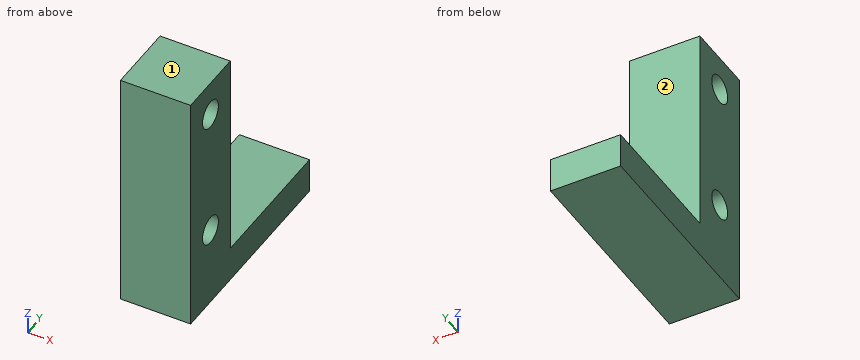
```python
from build123d import *

# Parameters (mm, degrees)
PAD_DEPTH    = 20
SKETCH001_R  = 4
POCKET_DEPTH = 20


with BuildPart() as part:
    # Sketch → Pad (new body)
    with BuildSketch(Plane.YZ):
        Polygon((-10, 35), (-10, -35), (50, -35), (50, -25), (10, -25), (10, 35), align=None)
    extrude(amount=PAD_DEPTH)

    # Sketch001 → Pocket (cut)
    with BuildSketch(Plane.YZ.offset(20)):
        with Locations((0, 25)):
            Circle(SKETCH001_R)
        with Locations((0, -12)):
            Circle(SKETCH001_R)
    extrude(amount=-POCKET_DEPTH, mode=Mode.SUBTRACT)


solid = part.part
```
Verification items for the finished model (mm, model axes). Face numbers are marked on the shaded views. A direction names the side the tool comes from. Give positions to 0.01 mm unless a question says otherwise; leave off trailing zeros. Loops run counter-clockwise (first coordinate to the right, second up) from the corner with the lowest first, then second, coordinate; pieces in that order, holes last.
1. Section check A-A, the plane y = 0. Enter the section's corners in (x, z).
2. Section check C-C, the plane x = 2.25. Enter the section's corners in (y, z).
3. Section check B-B, the plane z = 25. Enter the section's corners in (x, y).
4. Go/stop test with flat-tipped pins: pin 1 Ø6 at (x, y) = (11, 34) entering from +Z; pin 2 Ø10.5 at (y, z) = (0, -12) entering from -X; pin 3 Ø10 at (x, z) = (13, 7) entering from +Y. Record where each tip stops, or that it passes through.
5. Section check D-D, the plane z = 10.5. Enter the section's corners in (x, y), then the cut area to 3 significant figures.
6. Thickness scan on line 1 (Z direction, x = 15.5, y = 0); line 2 (Z direction, x = 13.25, y = -2.5); line 3 (Z direction, x = 4.25, y = 14). Record the ranges inside material, lowest first.
7. Set-up check for the marked faces 1 and 2: record each of +Z, -Z, +X, -X, +Y, -Y from which the full face is reachable in a straight line by a thin tool's end or side.
Geometry says:
1. outline: (0, -35) - (20, -35) - (20, -16) - (0, -16) - close; (0, -8) - (20, -8) - (20, 21) - (0, 21) - close; (0, 29) - (20, 29) - (20, 35) - (0, 35) - close
2. outline: (-10, -35) - (50, -35) - (50, -25) - (10, -25) - (10, 35) - (-10, 35) - close; hole circle Ø8 at (0, -12); hole circle Ø8 at (0, 25)
3. outline: (0, -10) - (20, -10) - (20, -4) - (0, -4) - close; (0, 4) - (20, 4) - (20, 10) - (0, 10) - close
4. pin 1: stops at z = -25
4. pin 2: stops at x = 0
4. pin 3: stops at y = 10
5. outline: (0, -10) - (20, -10) - (20, 10) - (0, 10) - close
5. area: 400 mm2
6. line 1: z = -35 to -16, -8 to 21, 29 to 35
6. line 2: z = -35 to -15.12, -8.88 to 21.88, 28.12 to 35
6. line 3: z = -35 to -25
7. face 1: +Z, +X, -X, +Y, -Y
7. face 2: +Z, +X, -X, +Y
